Autodesk Inventor part; units mm, degrees
ref_plane "YZ Plane" through (0, 0, 0) normal (1, 0, 0) x (0, 1, 0)
ref_plane "XZ Plane" through (0, 0, 0) normal (0, 1, 0) x (-1, 0, 0)
ref_plane "XY Plane" through (0, 0, 0) normal (0, 0, 1) x (1, 0, 0)
sketch "Sketch1" plane through (0, 0, 0) normal (0, 0, 1) x (1, 0, 0)
  circle A0 centre (-377.9563, 151.9963) radius 4.445
  circle A1 centre (-272.2465, 81.6053) radius 4.445
  circle A2 centre (-409.6686, 173.1136) radius 4.445
  line L0 (-413.1881, 167.8282) -> (-275.7661, 76.3199)
  arc A3 (-406.1491, 178.399) -> (-413.1881, 167.8282) centre (-409.6686, 173.1136) ccw
  line L1 (-268.727, 86.8907) -> (-406.1491, 178.399)
  arc A4 (-275.7661, 76.3199) -> (-268.727, 86.8907) centre (-272.2465, 81.6053) ccw
  circle A5 centre (-358.9063, 119.0008) radius 4.445 construction
  point P0 (0, 0)
  dimension "d0" = 8.89
  dimension "d1" = 8.89
  dimension "d2" = 8.89
  dimension "d3" = 8.89
extrude "Extrusion1" add sketch "Sketch1" along normal blind 3.175
equation "\"d0\" = d3"
equation "\"d1\" = d3"
equation "\"d2\" = d3"
The listing builds one solid part. Answer for the finished solid, in the listing's coordinates (mm). Round coordinates to 2 decimals unless told otherwise and drop trailing zeros. Write each loop counter-clockwise with the first axis right and the second up, starting at its lowest first coordinate (ties: lowest second). Pieces come first, ordered by that corner, then holes. Notation, with made-up numbers: (-21.75, 89) -> (22.25, 89) arc R31 ccw to (22.25, 118) -> close; hole circle Ø7 at (33.5, 83). An arc over 180 degrees is marked (long way). Use CSV: the item, a comma, the result in double quotes. Start each with the question number.
(1) Section C-C on y = 110 is taken. Give the vertices of the cut face in (x, z) (3 decimals), then the cut area to 3 significant figures.
(2) Consider L1, parallel to Y at x = -382, z = 0.85; L2, parallel to X at y = 83.5, z = 2.6; L3, parallel to Y at x = -275, z = 2.3. Determine where each line is inside the solid, lowest interval first. Write a range as from..to.
(3) Section A-A on x = -375.5 is taken. Give the vertices of the cut face in (y, z) (3 decimals).
(4) Section B-B on z = 1.65 is taken. Give the vertices of the cut face in (x, y) (1 decimal).
(5) The mould has two halves that part along X. Classify faces 1 (the face through (-415.03, 176.516, 1.565)), 2 (the face through (-341, 128, 0)), 3 (the face through (-272.83, 77.2, 1.57)), 4 (the face through (-412.945, 170.109, 1.565)): released by +X, released by -X, zero draft, split by the parting line, or undercut.
(6) Each of these flat-tipped pins is pushed along its axis until it touches: pin 1 (1 mm diameter, centred on x = -338.5, z = 2, fed in from +Y); pin 2 (1 mm diameter, centred on x = -313.5, y = 119.5, fed in from +Z); pin 3 (1.5 mm diameter, centred on y = 138, z = 2.5, fed in from +X). Where does it stop, or does it pass through?
A:
1,outline,"(-326.345, 0) -> (-303.431, 0) -> (-303.431, 3.175) -> (-326.345, 3.175) -> close"
1,area,"72.8 mm²"
2,L1,"y = 147.06..150.15, 153.84..162.32"
2,L2,"x = -286.55..-276.27, -268.23..-266.19"
2,L3,"y = 75.88..78.12, 85.09..91.07"
3,outline,"(142.732, 0) -> (148.292, 0) -> (148.292, 3.175) -> (142.732, 3.175) -> close; (155.701, 0) -> (157.99, 0) -> (157.99, 3.175) -> (155.701, 3.175) -> close"
4,outline,"(-413.2, 167.8) -> (-275.8, 76.3) arc R6.4 ccw to (-268.7, 86.9) -> (-406.1, 178.4) arc R6.3 ccw to start; hole circle Ø8.9 at (-409.7, 173.1); hole circle Ø8.9 at (-378, 152); hole circle Ø8.9 at (-272.2, 81.6)"
5,face 1,"split by the parting line"
5,face 2,"zero draft"
5,face 3,"undercut"
5,face 4,"undercut"
6,pin 1,"stops at y = 133.68"
6,pin 2,"passes through"
6,pin 3,"stops at x = -344.35"
